Read the model definition and answer for the solid it produces. Units are mm, in the model's axes. A direction names the side the tool comes from. Coordinates: 2 decimals unless noted, no trailing zeros. Loops run counter-clockwise (first coordinate to the right, second up) from the corner with the lowest first, then second, coordinate; pieces in that order, holes last. Notation, with made-up numbers: M 14.25,-3 L 53.25,-3 A33 ccw 53.25,29 Z; hole C 10.25,-8.5 d11. An arc over 180 degrees is marked long. Use one line per item in the form item = value. Start each with the question number.
1. A tool of negligible diameter and unlimited length cuts with its end or side. For faces 5 (the flat face through (47.5, 71, 38)), 6 (the flat face through (0, -60, 49)), 7 (the flat face through (-40, -10, 62)), from which of +Z, -Z, +X, -X, +Y, -Y can it reach the whole face along a straight path? Write none if from no direction.
2. The part is cut by section D-D (x = 66). Give the vertices of the cut face in (y, z), plus the area to 3 significant figures.
3. Flat-ended cylindrical pins translate along their axes: pin 1 (10 mm diameter, centred on x = -86, z = -4.5, fed in from +Y); pin 2 (1 mm diameter, centred on y = -56.5, z = 33, fed in from -X); pin 3 (12 mm diameter, centred on y = -4.5, z = 24.5, fed in from -X). Find the tip coordinate at first contact, or state that the pin passes through.
4. The part is cut by section A-A (z = 72.5). Give the vertices of the cut face in (x, y).
5. The part is cut by section B-B (x = -0.5). Give the vertices of the cut face in (y, z).
6. For a pull along Z with two mould halves and no side action, classify faces 1 (the cylindrical face through (-104.93, 2.17, 0.24)), 2 (the flat face through (85, -1, 62)), 3 (the cylindrical face through (1, -49, -12)), 4 (the cylindrical face through (18.11, -67.4, 89.55)) as released by +Z, released by -Z, zero draft, split by the parting line, or undercut.
7. The part is cut by section C-C (x = -26). Give the vertices of the cut face in (y, z).
8. Find the intervals of material crossed by probe 1 along Z at (x, y) = (-105.25, 0); probe 2 along X at (y, z) = (2, 42); probe 3 along Y at (x, z) = (-32, 48.5), in increasing order. Write a range as [from, to].
from build123d import *

# Parameters (mm, degrees)
F0_W           = 200
F0_H           = 120
F1_DEPTH       = 100
F2_T           = -15
F3_W           = 230
F3_H           = 150
F3_W_2         = 170
F3_H_2         = 90
F4_DEPTH       = 20
F5_W           = 200
F5_H           = 180
F6_DEPTH       = 20
F7_W           = 100
F7_H           = 10
F8_DEPTH       = 200
F9_R           = 5
F11_DEPTH      = 75
F11_DEPTH_BACK = 75
F12_DEPTH      = 45
F12_DEPTH_BACK = 45
F13_R          = 22.5
F14_DEPTH      = 200
F14_DEPTH_BACK = 200
F15_R          = 10
F19_DEPTH      = 7.5
F19_DEPTH_BACK = 7.5
F21_DEPTH      = 7.5
F21_DEPTH_BACK = 7.5
F22_DEPTH      = 200
F22_DEPTH_BACK = 200
F23_DEPTH      = 10
F24_R          = 10
F24_R_2        = 5
F25_DEPTH      = 10
F26_DEPTH      = 25
F27_R          = 15
F27_R_2        = 10
F28_DEPTH      = 5
F29_DEPTH      = 25
F30_W          = 70
F30_H          = 20
F31_DEPTH      = 115
F32_DEPTH      = 25
F32_DEPTH_BACK = 25


with BuildPart() as f1:
    # F0 (on Top) → F1 (new body)
    with BuildSketch(Plane.XY):
        Rectangle(F0_W, F0_H)
    extrude(amount=F1_DEPTH)

    # F2
    f2_openings = [f1.faces().sort_by_distance(p)[0] for p in [
        (0, 0, 100),
    ]]
    offset(amount=F2_T, openings=f2_openings)

    # F3 (on face) → F4 (join)
    with BuildSketch(Plane.XY.offset(100)):
        Rectangle(F3_W, F3_H)
        Rectangle(F3_W_2, F3_H_2, mode=Mode.SUBTRACT)
    extrude(amount=F4_DEPTH)

    # F5 (on face) → F6 (join)
    with BuildSketch(Plane(origin=(0, 0, 0), x_dir=(1, 0, 0), z_dir=(0, 0, -1))):
        Rectangle(F5_W, F5_H)
    extrude(amount=F6_DEPTH)

    # F7 (on face) → F8 (cut)
    with BuildSketch(Plane(origin=(-100, 0, 0), x_dir=(0, -1, 0), z_dir=(-1, 0, 0))):
        with Locations((0, -15)):
            Rectangle(F7_W, F7_H)
    extrude(amount=-F8_DEPTH, mode=Mode.SUBTRACT)

    # F9
    f9_edges = [f1.edges().sort_by_distance(p)[0] for p in [
        (0, -50, -10),
        (0, 50, -10),
    ]]
    fillet(f9_edges, radius=F9_R)

    # F10 (on Front) → F11 (join, two sides)
    with BuildSketch(Plane.XZ) as f11_sk:
        with BuildLine():
            Line((-2.5, 120), (-77.5, 120))
            ThreePointArc((-77.5, 120), (-40, 82.5), (-2.5, 120))
        make_face()
        with BuildLine():
            Line((77.5, 120), (2.5, 120))
            ThreePointArc((2.5, 120), (40, 82.5), (77.5, 120))
        make_face()
    extrude(amount=F11_DEPTH)
    extrude(f11_sk.sketch, amount=-F11_DEPTH_BACK)

    # F10 (on Front) → F12 (cut, two sides)
    with BuildSketch(Plane.XZ) as f12_sk:
        with BuildLine():
            Line((-2.5, 120), (-77.5, 120))
            ThreePointArc((-77.5, 120), (-40, 82.5), (-2.5, 120))
        make_face()
        with BuildLine():
            Line((77.5, 120), (2.5, 120))
            ThreePointArc((2.5, 120), (40, 82.5), (77.5, 120))
        make_face()
    extrude(amount=F12_DEPTH, mode=Mode.SUBTRACT)
    extrude(f12_sk.sketch, amount=-F12_DEPTH_BACK, mode=Mode.SUBTRACT)

    # F13 (on Front) → F14 (cut, two sides)
    with BuildSketch(Plane.XZ) as f14_sk:
        with Locations((-40, 120)):
            Circle(F13_R)
        with Locations((40, 120)):
            Circle(F13_R)
    extrude(amount=-F14_DEPTH, mode=Mode.SUBTRACT)
    extrude(f14_sk.sketch, amount=F14_DEPTH_BACK, mode=Mode.SUBTRACT)

    # F15
    f15_edges = [f1.edges().sort_by_distance(p)[0] for p in [
        (0, -90, 0),
        (0, 90, 0),
    ]]
    fillet(f15_edges, radius=F15_R)

    # F18 (on offset) → F19 (join, two sides)
    with BuildSketch(Plane.YZ.offset(40)) as f19_sk:
        Polygon((75, 82.5), (72.1370113349, 100), (60, 100), (60, 82.5), align=None)
        Polygon((89.8688040333, -8.3854700523), (75, 82.5), (60, 82.5), (60, -8.3854700523), align=None)
        Polygon((-60, 100), (-72.1370113349, 100), (-89.8688040333, -8.3854700523), (-60, -8.3854700523), align=None)
    extrude(amount=F19_DEPTH)
    extrude(f19_sk.sketch, amount=-F19_DEPTH_BACK)

    # F20 (on offset) → F21 (join, two sides)
    with BuildSketch(Plane.YZ.offset(-40)) as f21_sk:
        Polygon((89.8688040333, -8.3854700523), (72.1370113349, 100), (60, 100), (60, -8.3854700523), align=None)
        Polygon((-89.8688040333, -8.3854700523), (-60, -8.3854700523), (-60, 100), (-72.1370113349, 100), align=None)
    extrude(amount=F21_DEPTH)
    extrude(f21_sk.sketch, amount=-F21_DEPTH_BACK)

    # F13 (on Front) → F22 (cut, two sides)
    with BuildSketch(Plane.XZ) as f22_sk:
        with Locations((-40, 120)):
            Circle(F13_R)
        with Locations((40, 120)):
            Circle(F13_R)
    extrude(amount=-F22_DEPTH, mode=Mode.SUBTRACT)
    extrude(f22_sk.sketch, amount=F22_DEPTH_BACK, mode=Mode.SUBTRACT)

    # F23 (cut): a face of the model
    f23_faces = [f1.faces().sort_by_distance(p)[0] for p in [
        (0, 0, 15),
    ]]
    extrude(f23_faces, amount=-F23_DEPTH, mode=Mode.SUBTRACT)

    # F24 (on face) → F25 (join)
    with BuildSketch(Plane(origin=(-100, 0, 0), x_dir=(0, -1, 0), z_dir=(-1, 0, 0))):
        with Locations((0, 10)):
            Circle(F24_R)
        with Locations((0, 10)):
            Circle(F24_R_2, mode=Mode.SUBTRACT)
    extrude(amount=F25_DEPTH)

    # F26 (cut): a face of the model
    f26_faces = [f1.faces().sort_by_distance(p)[0] for p in [
        (-100, 0, 10),
    ]]
    extrude(f26_faces, amount=-F26_DEPTH, mode=Mode.SUBTRACT)

    # F27 (on face) → F28 (join)
    with BuildSketch(Plane.YZ.offset(100)):
        with Locations((0, 25)):
            Circle(F27_R)
        with Locations((0, 25)):
            Circle(F27_R_2, mode=Mode.SUBTRACT)
    extrude(amount=F28_DEPTH)

    # F29 (cut): a face of the model
    f29_faces = [f1.faces().sort_by_distance(p)[0] for p in [
        (100, 0, 25),
    ]]
    extrude(f29_faces, amount=-F29_DEPTH, mode=Mode.SUBTRACT)

    # F30 (on face) → F31 (join, through all)
    with BuildSketch(Plane.XY.offset(5)):
        with Locations((-40, 0)):
            Rectangle(F30_W, F30_H)
    extrude(amount=F31_DEPTH)

    # F13 (on Front) → F32 (cut, two sides)
    with BuildSketch(Plane.XZ) as f32_sk:
        with Locations((-40, 120)):
            Circle(F13_R)
        with Locations((40, 120)):
            Circle(F13_R)
    extrude(amount=-F32_DEPTH, mode=Mode.SUBTRACT)
    extrude(f32_sk.sketch, amount=F32_DEPTH_BACK, mode=Mode.SUBTRACT)


solid = f1.part
Computed values:
q1.face_5 = +X, +Y
q1.face_6 = -Y
q1.face_7 = +Z
q2.outline = M -90,-20 L -50,-20 L -50,-15 A5 cw -45,-10 L 45,-10 A5 cw 50,-15 L 50,-20 L 90,-20 L 90,-10 A10 ccw 80,0 L 60,0 L 60,92.98 L 75,92.98 L 75,120 L 45,120 L 45,5 L -45,5 L -45,120 L -75,120 L -75,92.98 L -60,92.98 L -60,0 L -80,0 A10 ccw -90,-10 Z
q2.area = 7,430 mm²
q3.pin_1 = 89.99
q3.pin_2 = -100
q3.pin_3 = -110
q4.outline = M -100,-60 L -47.5,-60 L -47.5,-76.64 L -32.5,-76.64 L -32.5,-60 L 32.5,-60 L 32.5,-76.64 L 47.5,-76.64 L 47.5,-60 L 100,-60 L 100,60 L 47.5,60 L 47.5,76.64 L 32.5,76.64 L 32.5,60 L -32.5,60 L -32.5,76.64 L -47.5,76.64 L -47.5,60 L -100,60 Z; M -75,-10 L -5,-10 L -5,10 L -75,10 Z; hole M -85,-45 L 85,-45 L 85,45 L -85,45 Z
q5.outline = M -90,-20 L -50,-20 L -50,-15 A5 cw -45,-10 L 45,-10 A5 cw 50,-15 L 50,-20 L 90,-20 L 90,-10 A10 ccw 80,0 L 60,0 L 60,100 L 75,100 L 75,120 L 45,120 L 45,5 L -45,5 L -45,120 L -75,120 L -75,100 L -60,100 L -60,0 L -80,0 A10 ccw -90,-10 Z
q6.face_1 = undercut
q6.face_2 = zero draft
q6.face_3 = released by -Z
q6.face_4 = undercut
q7.outline = M -90,-20 L -50,-20 L -50,-15 A5 cw -45,-10 L 45,-10 A5 cw 50,-15 L 50,-20 L 90,-20 L 90,-10 A10 ccw 80,0 L 60,0 L 60,85.21 L 75,85.21 L 75,102.39 L 45,102.39 L 45,5 L 10,5 L 10,102.39 L -10,102.39 L -10,5 L -45,5 L -45,102.39 L -75,102.39 L -75,85.21 L -60,85.21 L -60,0 L -80,0 A10 ccw -90,-10 Z
q8.probe_1 = [0, 5], [15, 20], [100, 120]
q8.probe_2 = [-100, -85], [-75, -5], [85, 100]
q8.probe_3 = [-60, -45], [-10, 10], [45, 60]
